Input: part model. Units: mm. Frame: model coordinates. A direction names the side the tool comes from. Round coordinates to 2 decimals unless told otherwise and drop trailing zeros. Loops run counter-clockwise (first coordinate to the right, second up) from the corner with the lowest first, then second, coordinate; pieces in that order, holes last. Notation, with made-up numbers: (42, -0.5) -> (46, -0.5) arc R11 ccw to (46, 15.5) -> close; hole circle Ø7 at (57, -37). An arc over 180 degrees is marked (long way). Answer in a Markdown table with one row per item. Add a question column.
Q1. Section B-B, the plane z = 10. Output: boundary loops of the cut face in (x, y), and give its area (3 significant figures).
Q2. Section A-A, the plane y = 81. Output: boundary loops of the cut face in (x, z), and give its area (3 significant figures).
Q3. Mould query, pull axis X, two halves, no side actions, for faces 1 (the face through (-105.941, 84, 10)), 2 (the face through (-55, 92.09, 10)), 3 (the face through (-182.821, 16, 10)). Classes: pulls with the +X half, pulls with the -X half, needs draft (parallel to the pull), parting line crosses it, or undercut.
Q4. Pin query (flat end, axial travel): pin 1 (10.5 mm diameter, centred on x = -16, z = 13.5, fed in from +Y); pin 2 (5 mm diameter, centred on x = -68.5, z = 10.5, fed in from +Y); pin 3 (4 mm diameter, centred on x = -100, z = 13.5, fed in from +Y). Return the tip coordinate at first contact, or that it passes through.
Q5. Ray query, L1, parallel to X at y = 73, z = 7; L2, parallel to X at y = 84.5, z = 8.75; L3, parallel to Y at x = -101.5, z = 4.75. Return the intervals inside material, ascending. Write a range as from..to.
Q6. Reachability of faces 4 (the face through (-20.664, 84, 10)), 5 (the face through (-59, -57.91, 10)) from +Z, -Z, +X, -X, +Y, -Y: full face, straight path, thin tool, end or side. Return the list, or none.
```python
from build123d import *

# Parameters (mm, degrees)
BOSS_EXTRUDE1_DEPTH = 20
SKETCH5_R           = 5.25
CUT_EXTRUDE4_DEPTH  = 20
SKETCH6_W           = 13
SKETCH6_H           = 13
CUT_EXTRUDE5_DEPTH  = 15.5
SKETCH7_W           = 13
SKETCH7_H           = 13
CUT_EXTRUDE6_DEPTH  = 15.5
SKETCH8_W           = 300
SKETCH8_H           = 102
BOSS_EXTRUDE2_DEPTH = 20
CUT_EXTRUDE7_START  = -150
SKETCH9_W           = 47.842391085
SKETCH9_H           = 20
CUT_EXTRUDE7_DEPTH  = 150


with BuildPart() as part:
    # Sketch1 → Boss-Extrude1 (new body)
    with BuildSketch(Plane.XY):
        Polygon((-107.821386225, 92.09039548), (-7.821386225, 92.09039548), (117.178613775, 92.09039548), (117.178613775, 44.09039548), (-7.821386225, 44.09039548), (-107.821386225, 44.09039548), (-182.821386225, 44.09039548), (-182.821386225, 92.09039548), align=None)
    extrude(amount=BOSS_EXTRUDE1_DEPTH)

    # Sketch5 → Cut-Extrude4 (cut)
    with BuildSketch(Plane(origin=(0, 92.09039548, 0), x_dir=(1, 0, 0), z_dir=(0, 1, 0))):
        with Locations(Location((-66.321386225, -10, 0), (0, 0, 180))):
            Circle(SKETCH5_R)
        with Locations(Location((-47.321386225, -10, 0), (0, 0, 180))):
            Circle(SKETCH5_R)
    extrude(amount=-CUT_EXTRUDE4_DEPTH, mode=Mode.SUBTRACT)

    # Sketch6 → Cut-Extrude5 (cut)
    with BuildSketch(Plane(origin=(0, 92.09039548, 0), x_dir=(1, 0, 0), z_dir=(0, 1, 0))):
        with Locations((-99.441386225, -10.25)):
            Rectangle(SKETCH6_W, SKETCH6_H)
    extrude(amount=-CUT_EXTRUDE5_DEPTH, mode=Mode.SUBTRACT)

    # Sketch7 → Cut-Extrude6 (cut)
    with BuildSketch(Plane(origin=(0, 92.09039548, 0), x_dir=(1, 0, 0), z_dir=(0, 1, 0))):
        with Locations((-14.16377731, -10.25)):
            Rectangle(SKETCH7_W, SKETCH7_H)
    extrude(amount=-CUT_EXTRUDE6_DEPTH, mode=Mode.SUBTRACT)

    # Sketch8 → Boss-Extrude2 (add)
    with BuildSketch(Plane.XY.offset(20)):
        with Locations((-32.821386225, -6.90960452)):
            Rectangle(SKETCH8_W, SKETCH8_H)
    extrude(amount=-BOSS_EXTRUDE2_DEPTH)

    # Sketch9 → Cut-Extrude7 (cut)
    with BuildSketch(Plane(origin=(0, 92.09039548, 0), x_dir=(1, 0, 0), z_dir=(0, 1, 0)).offset(CUT_EXTRUDE7_START)):
        with Locations((93.257418233, -10)):
            Rectangle(SKETCH9_W, SKETCH9_H)
    extrude(amount=CUT_EXTRUDE7_DEPTH, mode=Mode.SUBTRACT)


solid = part.part
```
Answer block:
| question | item | result |
|---|---|---|
| 1 | outline | (-182.82, -57.91) -> (69.34, -57.91) -> (69.34, 92.09) -> (-7.66, 92.09) -> (-7.66, 76.59) -> (-20.66, 76.59) -> (-20.66, 92.09) -> (-42.07, 92.09) -> (-42.07, 72.09) -> (-52.57, 72.09) -> (-52.57, 92.09) -> (-61.07, 92.09) -> (-61.07, 72.09) -> (-71.57, 72.09) -> (-71.57, 92.09) -> (-92.94, 92.09) -> (-92.94, 76.59) -> (-105.94, 76.59) -> (-105.94, 92.09) -> (-182.82, 92.09) -> close |
| 1 | area | 37,000 mm^2 |
| 2 | outline | (-182.82, 0) -> (69.34, 0) -> (69.34, 20) -> (-182.82, 20) -> close; hole (-105.94, 3.75) -> (-92.94, 3.75) -> (-92.94, 16.75) -> (-105.94, 16.75) -> close; hole circle Ø10.5 at (-66.32, 10); hole circle Ø10.5 at (-47.32, 10); hole (-20.66, 3.75) -> (-7.66, 3.75) -> (-7.66, 16.75) -> (-20.66, 16.75) -> close |
| 2 | area | 4,530 mm^2 |
| 3 | face 1 | undercut |
| 3 | face 2 | needs draft |
| 3 | face 3 | pulls with the -X half |
| 4 | pin 1 | y = 92.09 |
| 4 | pin 2 | y = 72.09 |
| 4 | pin 3 | y = 76.59 |
| 5 | L1 | -182.82..-70.63, -62.01..-51.63, -43.01..69.34 |
| 5 | L2 | -182.82..-105.94, -92.94..-71.42, -61.22..-52.42, -42.22..-20.66, -7.66..69.34 |
| 5 | L3 | -57.91..76.59 |
| 6 | face 4 | +Y |
| 6 | face 5 | +Z, -Z, +X, -X, -Y |
